The listing builds one solid part. Answer for the finished solid, in the listing's coordinates (mm). A direction names the side the tool comes from. Coordinates: 2 decimals unless noted, no trailing zeros. Write each loop counter-clockwise with the first axis right and the second up, starting at its lowest first coordinate (ties: lowest second). Pieces come first, ordered by that corner, then holes.
(1) The part is cut by section A-A on z = 6. Determine the outline of the cut face in (x, y).
(2) Straight lines are drawn through the part: line 1 (Z direction, x = 1.75, y = 2.25); line 2 (Y direction, x = 21.5, z = 2.75); line 3 (X direction, y = 23.5, z = 8.5). For each, find the intervals that lie inside material, in ascending order.
(3) Which of the six approach directions +Z, -Z, +X, -X, +Y, -Y give full straight-line access (tool end or side, diameter ignored) to faces 1 (the flat face through (24, 18.8, 6)), 2 (the flat face through (15, 16, 6)), 3 (the flat face through (5, 3, 9.1))?
(4) Given P1, Ø2, axis at y = 14, z = 2.5, coming from the -X side; P2, Ø4, axis at y = 5.5, z = 7.5, coming from the +X side; P3, Ø2, axis at x = 8, z = 4.5, coming from the +Y side; P4, Ø4, axis at x = 5, z = 9.5, coming from the +Y side, each flat-ended and moving along its own axis, determine where each tip first touches the part or whether it passes through.
(5) The part is cut by section D-D on y = 22.5. Determine the outline of the cut face in (x, z).
(6) The part is cut by section C-C on x = 22.5. Determine the outline of the cut face in (y, z), plus the area to 3 significant figures.
(7) The part is cut by section B-B on y = 3. Determine the outline of the cut face in (x, z), plus the area to 3 significant figures.
from build123d import *

# Parameters (mm, degrees)
PAD_DEPTH    = 12
POCKET_DEPTH = 6


with BuildPart() as part:
    # Sketch → Pad (new body)
    with BuildSketch(Plane.XY):
        Polygon((0, 0), (21, 0), (21, 18.8), (27, 18.8), (27, 24.8), (15, 24.8), (15, 6), (0, 6), align=None)
    extrude(amount=PAD_DEPTH)

    # Sketch002 (on Face1 of Pad) → Pocket (cut)
    with BuildSketch(Plane.XZ):
        with BuildLine():
            Line((0, 9.1), (10, 9.1))
            ThreePointArc((10, 2.9), (13.1, 6), (10, 9.1))
            Line((10, 2.9), (0, 2.9))
            ThreePointArc((0, 9.1), (-3.1, 6), (0, 2.9))
        make_face()
    extrude(amount=-POCKET_DEPTH, mode=Mode.SUBTRACT)


solid = part.part
Model answer:
1. outline: (13.1, 0) - (21, 0) - (21, 18.8) - (27, 18.8) - (27, 24.8) - (15, 24.8) - (15, 6) - (13.1, 6) - close
2. line 1: z = 0 to 2.9, 9.1 to 12
2. line 2: y = 18.8 to 24.8
2. line 3: x = 15 to 27
3. face 1: +Z, -Z, +X, -Y
3. face 2: +Z, -Z, -X, +Y
3. face 3: -X, +Y, -Y
4. P1: stops at x = 15
4. P2: stops at x = 21
4. P3: passes through
4. P4: stops at y = 6
5. outline: (15, 0) - (27, 0) - (27, 12) - (15, 12) - close
6. outline: (18.8, 0) - (24.8, 0) - (24.8, 12) - (18.8, 12) - close
6. area: 72.0 mm2
7. outline: (0, 0) - (21, 0) - (21, 12) - (0, 12) - (0, 9.1) - (10, 9.1) arc R3.1 cw to (10, 2.9) - (0, 2.9) - close
7. area: 175 mm2
